```python
from build123d import *

# Parameters (mm, degrees)
CROQUIS1_W              = 36
CROQUIS1_H              = 27
SALIENTE_EXTRUIR1_DEPTH = 10
CROQUIS2_R              = 1.5
CORTAR_EXTRUIR1_DEPTH   = 5
CORTAR_EXTRUIR2_DEPTH   = 36


with BuildPart() as part:
    # Croquis1 → Saliente-Extruir1 (new body)
    with BuildSketch(Plane(origin=(0, 0, 0), x_dir=(1, 0, 0), z_dir=(0, 1, 0))):
        with Locations((18, 13.5)):
            Rectangle(CROQUIS1_W, CROQUIS1_H)
    extrude(amount=SALIENTE_EXTRUIR1_DEPTH)

    # Croquis2 → Cortar-Extruir1 (cut)
    with BuildSketch(Plane(origin=(0, 10, 0), x_dir=(1, 0, 0), z_dir=(0, 1, 0))):
        with Locations((10.5, 23.52014925)):
            Circle(CROQUIS2_R)
        with Locations((25.499986467, 23.5)):
            Circle(CROQUIS2_R)
        with Locations((10.5, 3.52014925)):
            Circle(CROQUIS2_R)
        with Locations((25.499986467, 3.5)):
            Circle(CROQUIS2_R)
    extrude(amount=-CORTAR_EXTRUIR1_DEPTH, mode=Mode.SUBTRACT)

    # Croquis3 → Cortar-Extruir2 (cut)
    with BuildSketch(Plane(origin=(36, 0, 0), x_dir=(0, 0, -1), z_dir=(1, 0, 0))):
        Polygon((7.5, 0), (19.5, 0), (19.5, 1.3), (17.8, 1.3), (17.8, 3.1), (19.5, 3.1), (19.5, 4.5), (7.5, 4.5), (7.5, 3.1), (9.2, 3.1), (9.2, 1.3), (7.5, 1.3), align=None)
    extrude(amount=-CORTAR_EXTRUIR2_DEPTH, mode=Mode.SUBTRACT)


solid = part.part
```
The listing builds one solid part. Answer for the finished solid, in the listing's coordinates (mm). A direction names the side the tool comes from. Coordinates: 2 decimals unless noted, no trailing zeros. Write each loop counter-clockwise with the first axis right and the second up, starting at its lowest first coordinate (ties: lowest second). Pieces come first, ordered by that corner, then holes. Notation, with made-up numbers: (3, 10) - (27, 10) arc R25 ccw to (27, 22) - close; hole circle Ø7 at (65.5, -39.5). An arc over 180 degrees is marked (long way). Return JSON: item names as keys, results as strings. Group by question number.
Q1. The part is cut by section B-B on x = 10.5. Write down the section's boundary in (y, z), and give its area (3 significant figures).
Q2. Flat-ended cylindrical pins translate along their axes: pin 1 Ø0.8 at (x, z) = (13, -18.5) entering from -Y; pin 2 Ø2.5 at (x, z) = (25.5, -23.5) entering from +Y; pin 3 Ø1 at (x, z) = (30.5, -14) entering from -Y. Find the tip coordinate at first contact, or state that the pin passes through.
Q3. The part is cut by section D-D on x = 15.5. Write down the section's boundary in (y, z).
Q4. The part is cut by section A-A on y = 2. Write down the section's boundary in (x, z).
Q5. The part is cut by section C-C on y = 3.75. Write down the section's boundary in (x, z).
Q6. Find the intervals of material crossed by line 1 along Z through (x, y) = (10.5, 7.95); line 2 along X through (y, z) = (7.4, -3.5); line 3 along Z through (x, y) = (30.5, 1.25), in increasing order. Write a range as [from, to].
Q7. Which of the six approach directions +Z, -Z, +X, -X, +Y, -Y give full straight-line access (tool end or side, diameter ignored) to faces 4 (the flat face through (10, 5, -24)), 5 (the flat face through (18, 1, -19.5)), 6 (the flat face through (18, 4, -7.5)), 7 (the flat face through (36, 6, -13)), 8 (the flat face through (18, 0, -4))?
Q8. For a pull along Y with two mould halves and no side action, classify faces 1 (the flat face through (18, 4.5, -14)), 2 (the flat face through (18, 5, -27)), 3 (the flat face through (18, 10, -14)) as +Y half, -Y half, draft (parallel to the pull), parting line (faces both ways), or undercut.
Evaluation:
{
 "1": {"outline": "(0, -27) - (10, -27) - (10, -25.02) - (5, -25.02) - (5, -22.02) - (10, -22.02) - (10, -5.02) - (5, -5.02) - (5, -2.02) - (10, -2.02) - (10, 0) - (0, 0) - (0, -7.5) - (1.3, -7.5) - (1.3, -9.2) - (3.1, -9.2) - (3.1, -7.5) - (4.5, -7.5) - (4.5, -19.5) - (3.1, -19.5) - (3.1, -17.8) - (1.3, -17.8) - (1.3, -19.5) - (0, -19.5) - close", "area": "192 mm2"},
 "2": {"pin 1": "stops at y = 1.3", "pin 2": "stops at y = 5", "pin 3": "stops at y = 4.5"},
 "3": {"outline": "(0, -27) - (10, -27) - (10, 0) - (0, 0) - (0, -7.5) - (1.3, -7.5) - (1.3, -9.2) - (3.1, -9.2) - (3.1, -7.5) - (4.5, -7.5) - (4.5, -19.5) - (3.1, -19.5) - (3.1, -17.8) - (1.3, -17.8) - (1.3, -19.5) - (0, -19.5) - close"},
 "4": {"outline": "(0, -27) - (36, -27) - (36, -17.8) - (0, -17.8) - close; (0, -9.2) - (36, -9.2) - (36, 0) - (0, 0) - close"},
 "5": {"outline": "(0, -27) - (36, -27) - (36, -19.5) - (0, -19.5) - close; (0, -7.5) - (36, -7.5) - (36, 0) - (0, 0) - close"},
 "6": {"line 1": "z = [-27, -25.02], [-22.02, -5.02], [-2.02, 0]", "line 2": "x = [0, 9], [12, 24], [27, 36]", "line 3": "z = [-27, -19.5], [-7.5, 0]"},
 "7": {"face 4": "+Y", "face 5": "+X, -X, -Y", "face 6": "+X, -X", "face 7": "+Z, -Z, +X, +Y, -Y", "face 8": "+Z, -Z, +X, -X, -Y"},
 "8": {"face 1": "undercut", "face 2": "draft", "face 3": "+Y half"}
}
